```python
from build123d import *
from OCP.BRepFilletAPI import BRepFilletAPI_MakeChamfer

# Parameters (mm, degrees)
BOSS_EXTRUDE1_DEPTH = 30
SKETCH2_W           = 57
SKETCH2_H           = 22
CUT_EXTRUDE1_DEPTH  = 84.417744515
SKETCH4_R           = 8
SKETCH4_R_2         = 1.75
CUT_EXTRUDE2_DEPTH  = 79.315898929
SKETCH5_R           = 14
CUT_EXTRUDE3_DEPTH  = 37
SKETCH6_R           = 1.75
CUT_EXTRUDE4_DEPTH  = 60.307503952
CHAMFER1_SIZE       = 10
CHAMFER1_SIZE2      = 14.281480067
FILLET3_R           = 20
SKETCH11_W          = 2
SKETCH11_H          = 14.29
BOSS_EXTRUDE3_DEPTH = 12.7
CHAMFER2_SIZE       = 5
CHAMFER2_SIZE_2     = 13.025445323


with BuildPart() as part:
    # Sketch1 → Boss-Extrude1 (new body)
    with BuildSketch(Plane(origin=(0, 0, 0), x_dir=(1, 0, 0), z_dir=(0, 1, 0))):
        Polygon((0, 0), (0, -17.465), (-20, -17.465), (-20, -31.755), (45, -31.755), (45, 0), align=None)
        Polygon((0, 17.465), (0, 0), (45, 0), (45, 31.755), (-20, 31.755), (-20, 17.465), align=None)
    extrude(amount=BOSS_EXTRUDE1_DEPTH)

    # Sketch2 → Cut-Extrude1 (cut, through all)
    with BuildSketch(Plane.XY.offset(31.755)):
        with Locations((8.5, 19)):
            Rectangle(SKETCH2_W, SKETCH2_H)
    extrude(amount=-CUT_EXTRUDE1_DEPTH, mode=Mode.SUBTRACT)

    # Sketch4 → Cut-Extrude2 (cut, through all)
    with BuildSketch(Plane(origin=(45, 0, 0), x_dir=(0, 0, -1), z_dir=(1, 0, 0))):
        with Locations((0, 15.135)):
            Circle(SKETCH4_R)
        with Locations((-7.778174593, 22.683263808)):
            Circle(SKETCH4_R_2)
        with Locations((7.778174593, 22.913174593)):
            Circle(SKETCH4_R_2)
        with Locations((7.778174593, 7.356825407)):
            Circle(SKETCH4_R_2)
        with Locations((-7.778174593, 7.356825407)):
            Circle(SKETCH4_R_2)
    extrude(amount=-CUT_EXTRUDE2_DEPTH, mode=Mode.SUBTRACT)

    # Sketch5 → Cut-Extrude3 (cut)
    with BuildSketch(Plane.ZY):
        with Locations((0, 15.135)):
            Circle(SKETCH5_R)
    extrude(amount=-CUT_EXTRUDE3_DEPTH, mode=Mode.SUBTRACT)

    # Sketch6 → Cut-Extrude4 (cut, through all)
    with BuildSketch(Plane(origin=(0, 8, 0), x_dir=(1, 0, 0), z_dir=(0, 1, 0))):
        with Locations(Location((-5, -20.465, 0), (0, 0, 270))):
            Circle(SKETCH6_R)
    cut_extrude4 = extrude(amount=-CUT_EXTRUDE4_DEPTH, mode=Mode.SUBTRACT)

    # Mirror1: Cut-Extrude4 across plane
    add(cut_extrude4.mirror(Plane.XY), mode=Mode.SUBTRACT)

    # Chamfer1: one chamfer whose edges measure the first distance from different faces: ONE call of the kernel's chamfer builder (chamfer() names one face for all edges)
    chamfer1_edges_1 = [part.edges().sort_by_distance(p)[0] for p in [
        (37, 8, -21.900202363),
    ]]
    chamfer1_side_1 = [part.faces().sort_by_distance(p)[0] for p in [
        (10.623596069, 8, -22.684210572),
    ]]
    chamfer1_edges_2 = [part.edges().sort_by_distance(p)[0] for p in [
        (37, 8, 21.900202363),
    ]]
    chamfer1_side_2 = [part.faces().sort_by_distance(p)[0] for p in [
        (10.623596069, 8, 22.684210572),
    ]]
    chamfer1 = BRepFilletAPI_MakeChamfer(part.part.solid().wrapped)
    for e in chamfer1_edges_1:
        chamfer1.Add(CHAMFER1_SIZE, CHAMFER1_SIZE2, e.wrapped, chamfer1_side_1[0].wrapped)  # the first distance lies on this face
    for e in chamfer1_edges_2:
        chamfer1.Add(CHAMFER1_SIZE, CHAMFER1_SIZE2, e.wrapped, chamfer1_side_2[0].wrapped)  # the first distance lies on this face
    add(Compound.cast(chamfer1.Shape()), mode=Mode.REPLACE)

    # Fillet3
    fillet3_edges = [part.edges().sort_by_distance(p)[0] for p in [
        (41, 30, -31.755),
        (41, 30, 31.755),
    ]]
    fillet(fillet3_edges, radius=FILLET3_R)

    # Sketch11 → Boss-Extrude3 (add)
    with BuildSketch(Plane.XZ):
        with Locations((1, 24.61)):
            Rectangle(SKETCH11_W, SKETCH11_H)
        with Locations((1, -24.61)):
            Rectangle(SKETCH11_W, SKETCH11_H)
        with Locations((1, 0)):
            Rectangle(SKETCH11_W, SKETCH11_H)
    extrude(amount=BOSS_EXTRUDE3_DEPTH)

    # Chamfer2
    # the kernel refuses this chamfer: 13.025445323, 5 mm, written as the material it adds along each edge
    with BuildSketch(Plane(origin=(2, 0, -16.317868448), x_dir=(0.9956314177255227, 0.0933706594057566, 0), z_dir=(0, 0, 1))) as chamfer2_piece_1_section:
        Polygon((CHAMFER2_SIZE * 0.995631417726, -CHAMFER2_SIZE * 0.0933706594058), (-CHAMFER2_SIZE_2 * 0.0933706594091, -CHAMFER2_SIZE_2 * 0.995631417761), (0, 0), align=None)
    chamfer2_piece_1 = extrude(amount=48.072868448, mode=Mode.PRIVATE)
    chamfer2_piece_1 = split(chamfer2_piece_1, bisect_by=Plane(origin=(3.561931583, -4.37126632, 7.145), z_dir=(0, 0, -1)), keep=Keep.TOP, mode=Mode.PRIVATE)
    chamfer2_piece_1 = split(chamfer2_piece_1, bisect_by=Plane(origin=(3.561931583, -4.37126632, -7.145), z_dir=(0, 0, 1)), keep=Keep.TOP, mode=Mode.PRIVATE)
    chamfer2_piece_1 = split(chamfer2_piece_1, bisect_by=Plane(origin=(3.561931583, -12.7, 0), z_dir=(0, 1, 0)), keep=Keep.TOP, mode=Mode.PRIVATE)
    add(chamfer2_piece_1)
    with BuildSketch(Plane(origin=(2, 0, 17.465), x_dir=(0.9956314177255227, 0.0933706594057566, 0), z_dir=(0, 0, 1))) as chamfer2_piece_2_section:
        Polygon((CHAMFER2_SIZE * 0.995631417726, -CHAMFER2_SIZE * 0.0933706594058), (-CHAMFER2_SIZE_2 * 0.0933706594091, -CHAMFER2_SIZE_2 * 0.995631417761), (0, 0), align=None)
    chamfer2_piece_2 = extrude(amount=14.29, mode=Mode.PRIVATE)
    chamfer2_piece_2 = split(chamfer2_piece_2, bisect_by=Plane(origin=(3.561931583, -12.7, 24.61), z_dir=(0, 1, 0)), keep=Keep.TOP, mode=Mode.PRIVATE)
    add(chamfer2_piece_2)
    with BuildSketch(Plane(origin=(2, 0, 40.927868448), x_dir=(0.9956314177255227, 0.0933706594057566, 0), z_dir=(0, 0, -1))) as chamfer2_piece_3_section:
        Polygon((CHAMFER2_SIZE * 0.995631417726, CHAMFER2_SIZE * 0.0933706594058), (-CHAMFER2_SIZE_2 * 0.0933706594091, CHAMFER2_SIZE_2 * 0.995631417761), (0, 0), align=None)
    chamfer2_piece_3 = extrude(amount=48.072868448, mode=Mode.PRIVATE)
    chamfer2_piece_3 = split(chamfer2_piece_3, bisect_by=Plane(origin=(3.561931583, -4.37126632, 31.755), z_dir=(0, 0, -1)), keep=Keep.TOP, mode=Mode.PRIVATE)
    chamfer2_piece_3 = split(chamfer2_piece_3, bisect_by=Plane(origin=(3.561931583, -12.7, 24.61), z_dir=(0, 1, 0)), keep=Keep.TOP, mode=Mode.PRIVATE)
    chamfer2_piece_3 = split(chamfer2_piece_3, bisect_by=Plane(origin=(3.561931583, -4.37126632, 17.465), z_dir=(0, 0, 1)), keep=Keep.TOP, mode=Mode.PRIVATE)
    add(chamfer2_piece_3)
    with BuildSketch(Plane(origin=(2, 0, 7.145), x_dir=(0.9956314177255227, 0.0933706594057566, 0), z_dir=(0, 0, -1))) as chamfer2_piece_4_section:
        Polygon((CHAMFER2_SIZE * 0.995631417726, CHAMFER2_SIZE * 0.0933706594058), (-CHAMFER2_SIZE_2 * 0.0933706594091, CHAMFER2_SIZE_2 * 0.995631417761), (0, 0), align=None)
    chamfer2_piece_4 = extrude(amount=14.29, mode=Mode.PRIVATE)
    chamfer2_piece_4 = split(chamfer2_piece_4, bisect_by=Plane(origin=(3.561931583, -12.7, 0), z_dir=(0, 1, 0)), keep=Keep.TOP, mode=Mode.PRIVATE)
    add(chamfer2_piece_4)
    with BuildSketch(Plane(origin=(2, 0, 7.145), x_dir=(0.9956314177255227, 0.0933706594057566, 0), z_dir=(0, 0, -1))) as chamfer2_piece_5_section:
        Polygon((CHAMFER2_SIZE * 0.995631417726, CHAMFER2_SIZE * 0.0933706594058), (-CHAMFER2_SIZE_2 * 0.0933706594091, CHAMFER2_SIZE_2 * 0.995631417761), (0, 0), align=None)
    chamfer2_piece_5 = extrude(amount=48.072868448, mode=Mode.PRIVATE)
    chamfer2_piece_5 = split(chamfer2_piece_5, bisect_by=Plane(origin=(3.561931583, -4.37126632, -31.755), z_dir=(0, 0, 1)), keep=Keep.TOP, mode=Mode.PRIVATE)
    chamfer2_piece_5 = split(chamfer2_piece_5, bisect_by=Plane(origin=(3.561931583, -12.7, -24.61), z_dir=(0, 1, 0)), keep=Keep.TOP, mode=Mode.PRIVATE)
    chamfer2_piece_5 = split(chamfer2_piece_5, bisect_by=Plane(origin=(3.561931583, -4.37126632, -17.465), z_dir=(0, 0, -1)), keep=Keep.TOP, mode=Mode.PRIVATE)
    add(chamfer2_piece_5)
    with BuildSketch(Plane(origin=(2, 0, 16.317868448), x_dir=(0.9956314177255227, 0.0933706594057566, 0), z_dir=(0, 0, -1))) as chamfer2_piece_6_section:
        Polygon((CHAMFER2_SIZE * 0.995631417726, CHAMFER2_SIZE * 0.0933706594058), (-CHAMFER2_SIZE_2 * 0.0933706594091, CHAMFER2_SIZE_2 * 0.995631417761), (0, 0), align=None)
    chamfer2_piece_6 = extrude(amount=48.072868448, mode=Mode.PRIVATE)
    chamfer2_piece_6 = split(chamfer2_piece_6, bisect_by=Plane(origin=(3.561931583, -4.37126632, 7.145), z_dir=(0, 0, -1)), keep=Keep.TOP, mode=Mode.PRIVATE)
    chamfer2_piece_6 = split(chamfer2_piece_6, bisect_by=Plane(origin=(3.561931583, -4.37126632, -7.145), z_dir=(0, 0, 1)), keep=Keep.TOP, mode=Mode.PRIVATE)
    chamfer2_piece_6 = split(chamfer2_piece_6, bisect_by=Plane(origin=(3.561931583, -12.7, 0), z_dir=(0, 1, 0)), keep=Keep.TOP, mode=Mode.PRIVATE)
    add(chamfer2_piece_6)
    with BuildSketch(Plane(origin=(2, 0, -17.465), x_dir=(0.9956314177255227, 0.0933706594057566, 0), z_dir=(0, 0, -1))) as chamfer2_piece_7_section:
        Polygon((CHAMFER2_SIZE * 0.995631417726, CHAMFER2_SIZE * 0.0933706594058), (-CHAMFER2_SIZE_2 * 0.0933706594091, CHAMFER2_SIZE_2 * 0.995631417761), (0, 0), align=None)
    chamfer2_piece_7 = extrude(amount=14.29, mode=Mode.PRIVATE)
    chamfer2_piece_7 = split(chamfer2_piece_7, bisect_by=Plane(origin=(3.561931583, -12.7, -24.61), z_dir=(0, 1, 0)), keep=Keep.TOP, mode=Mode.PRIVATE)
    add(chamfer2_piece_7)


solid = part.part
```
For this review, take the finished solid that the model builds, in its own axes (mm). A direction names the side the tool comes from. Coordinates: 2 decimals unless noted, no trailing zeros. Order: outer loops, then holes, each group sorted by start corner. A loop starts at its lowest first (then second) coordinate and runs counter-clockwise, first axis right, second up. Notation, with made-up numbers: (11, -25) - (58, -25) arc R16 ccw to (58, -14) - close; hole circle Ø1 at (-3.75, 59). An arc over 180 degrees is marked (long way). Answer as a JSON object with one key per item and string values. Group by question number.
1. We need section D-D on y = 12. State the section outline as (x, z) points.
2. We need section C-C on y = -6. State the section outline as (x, z) points (3 decimals), then the cut area to 3 significant figures.
3. Clearance check with flat-ended pins moving along their axes: P1, Ø4, axis at x = -5, z = 20.465, coming from the -Y side; P2, Ø1, axis at y = 14, z = -23, coming from the -X side; P3, Ø4, axis at y = -8.5, z = -27.5, coming from the -X side; P4, Ø3, axis at y = 22.91, z = -7.78, coming from the +X side. State where each tip first meets the part, or that it passes through.
4. The part is to be moulded in two halves that separate along Y. For faces 1 (the flat face through (22, 0, 0)), 2 (the cylindrical face through (41.06, 7.43, -6.03)), 3 (the flat face through (2, -5, 17.465)), 4 (the cylindrical face through (41.056, 24.418, 8.006)), say which applies: pulls with the +Y half, pulls with the -Y half, needs draft (parallel to the pull), parting line crosses it, or undercut.
5. We need section B-B on z = 0. State the section outline as (x, y) points (3 decimals).
6. For probe 1 along Z at (x, y) = (40.5, 15); probe 2 along X at (y, z) = (15, -10); probe 3 along Z at (x, y) = (-1.5, 2) (3 decimals), list the stretches that pass through material, from the lowest coordinate up.
7. For faces 5 (the flat face through (3, 8, -24)), 6 (the flat face through (-10, 0, 25)), 7 (the flat face through (3, -5, -17.465)), list the 3-axis set-ups (+Z, -Z, +X, -X, +Y, -Y) from which the entire face can be reached by the end or side of a thin tool; tool diameter is ignored.
8. We need section A-A on x = -5. State the section outline as (y, z) points (3 decimals).
Final values:
{
 "1": {"outline": "(29.8, -31.65) - (45, -31.65) - (45, -7.36) - (37, -7.36) - (37, -13.64) - (29.8, -13.64) - close; (29.8, 13.64) - (37, 13.64) - (37, 7.36) - (45, 7.36) - (45, 31.65) - (29.8, 31.65) - close"},
 "2": {"outline": "(0, -31.755) - (4.697, -31.755) - (4.697, -17.465) - (0, -17.465) - close; (0, -7.145) - (4.697, -7.145) - (4.697, 7.145) - (0, 7.145) - close; (0, 17.465) - (4.697, 17.465) - (4.697, 31.755) - (0, 31.755) - close", "area": "201 mm²"},
 "3": {"P1": "y = 0", "P2": "x = 30.85", "P3": "x = 0", "P4": "through"},
 "4": {"face 1": "pulls with the -Y half", "face 2": "undercut", "face 3": "needs draft", "face 4": "undercut"},
 "5": {"outline": "(0, -12.7) - (2.125, -12.7) - (7, 0) - (45, 0) - (45, 7.135) - (37, 7.135) - (37, 1.135) - (0, 1.135) - close; (37, 23.135) - (45, 23.135) - (45, 30) - (37, 30) - close"},
 "6": {"probe 1": "-31.12 to -8, 8 to 31.12", "probe 2": "37 to 45", "probe 3": "-31.755 to -17.465, 17.465 to 31.755"},
 "7": {"face 5": "+Z, -Z, -X, +Y", "face 6": "+Z, -Z, -X, -Y", "face 7": "+X, -X, -Y"},
 "8": {"outline": "(0, -31.755) - (8, -31.755) - (8, -22.215) - (0, -22.215) - close; (0, -18.715) - (8, -18.715) - (8, -17.465) - (0, -17.465) - close; (0, 17.465) - (8, 17.465) - (8, 18.715) - (0, 18.715) - close; (0, 22.215) - (8, 22.215) - (8, 31.755) - (0, 31.755) - close"}
}
